```python
from build123d import *

# Parameters (mm, degrees)
BOSS_EXTRUDE1_DEPTH = 29.5
CUT_EXTRUDE1_DEPTH  = 27.5
SKETCH4_R           = 1.375
BOSS_EXTRUDE2_DEPTH = 6
CUT_EXTRUDE2_REACH  = 62
SKETCH5_W           = 8.5
SKETCH5_H           = 4
CUT_EXTRUDE3_REACH  = 64
SKETCH6_W           = 10
SKETCH6_H           = 6
BOSS_EXTRUDE3_DEPTH = 12
FILLET1_R           = 1


with BuildPart() as part:
    # Sketch1 → Boss-Extrude1 (new body)
    with BuildSketch(Plane(origin=(0, 0, 0), x_dir=(1, 0, 0), z_dir=(0, 1, 0))):
        with BuildLine():
            Line((-25, -31), (25, -31))
            ThreePointArc((25, -31), (28.535533906, -29.535533906), (30, -26))
            Line((30, -26), (30, 26))
            ThreePointArc((30, 26), (28.535533906, 29.535533906), (25, 31))
            Line((25, 31), (-25, 31))
            ThreePointArc((-25, 31), (-28.535533906, 29.535533906), (-30, 26))
            Line((-30, 26), (-30, -26))
            ThreePointArc((-30, -26), (-28.535533906, -29.535533906), (-25, -31))
        make_face()
    extrude(amount=BOSS_EXTRUDE1_DEPTH)

    # Sketch2 → Cut-Extrude1 (cut)
    with BuildSketch(Plane(origin=(0, 29.5, 0), x_dir=(1, 0, 0), z_dir=(0, 1, 0))):
        with BuildLine():
            Line((-25, -29), (25, -29))
            ThreePointArc((25, -29), (27.121320344, -28.121320344), (28, -26))
            Line((28, -26), (28, 26))
            ThreePointArc((28, 26), (27.121320344, 28.121320344), (25, 29))
            Line((25, 29), (-25, 29))
            ThreePointArc((-25, 29), (-27.121320344, 28.121320344), (-28, 26))
            Line((-28, 26), (-28, -26))
            ThreePointArc((-28, -26), (-27.121320344, -28.121320344), (-25, -29))
        make_face()
    extrude(amount=-CUT_EXTRUDE1_DEPTH, mode=Mode.SUBTRACT)

    # Sketch4 → Boss-Extrude2 (add)
    with BuildSketch(Plane(origin=(0, 2, 0), x_dir=(1, 0, 0), z_dir=(0, 1, 0))):
        with BuildLine():
            Line((-17.25, 23.25), (-17.25, 29))
            Line((-17.25, 29), (-25, 29))
            ThreePointArc((-25, 29), (-27.121320344, 28.121320344), (-28, 26))
            Line((-28, 26), (-28, 18.25))
            Line((-28, 18.25), (-22.25, 18.25))
            ThreePointArc((-22.25, 18.25), (-18.714466094, 19.714466094), (-17.25, 23.25))
        make_face()
        with Locations((-22.25, 23.25)):
            Circle(SKETCH4_R, mode=Mode.SUBTRACT)
        with BuildLine():
            Line((22.25, 18.25), (28, 18.25))
            Line((28, 18.25), (28, 26))
            ThreePointArc((28, 26), (27.121320344, 28.121320344), (25, 29))
            Line((25, 29), (17.25, 29))
            Line((17.25, 29), (17.25, 23.25))
            ThreePointArc((17.25, 23.25), (18.714466094, 19.714466094), (22.25, 18.25))
        make_face()
        with Locations((22.25, 23.25)):
            Circle(SKETCH4_R, mode=Mode.SUBTRACT)
        with BuildLine():
            Line((-25, -29), (-17.25, -29))
            Line((-17.25, -29), (-17.25, -23.25))
            ThreePointArc((-17.25, -23.25), (-18.714466094, -19.714466094), (-22.25, -18.25))
            Line((-22.25, -18.25), (-28, -18.25))
            Line((-28, -18.25), (-28, -26))
            ThreePointArc((-28, -26), (-27.121320344, -28.121320344), (-25, -29))
        make_face()
        with Locations((-22.25, -23.25)):
            Circle(SKETCH4_R, mode=Mode.SUBTRACT)
        with BuildLine():
            Line((28, -26), (28, -18.25))
            Line((28, -18.25), (22.25, -18.25))
            ThreePointArc((22.25, -18.25), (18.714466094, -19.714466094), (17.25, -23.25))
            Line((17.25, -23.25), (17.25, -29))
            Line((17.25, -29), (25, -29))
            ThreePointArc((25, -29), (27.121320344, -28.121320344), (28, -26))
        make_face()
        with Locations((22.25, -23.25)):
            Circle(SKETCH4_R, mode=Mode.SUBTRACT)
    extrude(amount=BOSS_EXTRUDE2_DEPTH)

    # Sketch5 → Cut-Extrude2 (cut, up to next)
    with BuildSketch(Plane.ZY.offset(30), mode=Mode.PRIVATE) as cut_extrude2_sk1:
        with Locations((-8.5, 18)):
            Rectangle(SKETCH5_W, SKETCH5_H)
    cut_extrude2_tool1 = extrude(cut_extrude2_sk1.sketch, amount=-CUT_EXTRUDE2_REACH, mode=Mode.PRIVATE) & part.part
    add(cut_extrude2_tool1.solids().sort_by_distance((-30, 18, -8.5))[0], mode=Mode.SUBTRACT)

    # Sketch6 → Cut-Extrude3 (cut, up to next)
    with BuildSketch(Plane(origin=(0, 0, -31), x_dir=(-1, 0, 0), z_dir=(0, 0, -1)), mode=Mode.PRIVATE) as cut_extrude3_sk1:
        with Locations((11.75, 19)):
            Rectangle(SKETCH6_W, SKETCH6_H)
    cut_extrude3_tool1 = extrude(cut_extrude3_sk1.sketch, amount=-CUT_EXTRUDE3_REACH, mode=Mode.PRIVATE) & part.part
    add(cut_extrude3_tool1.solids().sort_by_distance((-11.75, 19, -31))[0], mode=Mode.SUBTRACT)

    # Sketch7 → Boss-Extrude3 (add)
    with BuildSketch(Plane.ZY.offset(6)):
        Polygon((-29, 29.5), (-29, 26.5), (-27, 29.5), align=None)
    extrude(amount=-BOSS_EXTRUDE3_DEPTH)

    # Fillet1
    fillet1_edges = [part.edges().sort_by_distance(p)[0] for p in [
        (0, 0, -31),
        (28.535533906, 0, -29.535533906),
        (30, 0, 0),
        (28.535533906, 0, 29.535533906),
        (0, 0, 31),
        (-28.535533906, 0, 29.535533906),
        (-30, 0, 0),
        (-28.535533906, 0, -29.535533906),
    ]]
    fillet(fillet1_edges, radius=FILLET1_R)


solid = part.part
```
CAD build for the part. Positions are in the model's coordinates, mm. A direction names the side the tool comes from. Coordinates: 2 decimals unless noted, no trailing zeros. Order: outer loops, then holes, each group sorted by start corner. A loop starts at its lowest first (then second) coordinate and runs counter-clockwise, first axis right, second up.
(1) Saw through at C-C, the plane z = -11.5. Write the cut outline in (x, y), and give its area (3 significant figures).
Solution:
outline: (-30, 1) arc R1 ccw to (-29, 0) - (29, 0) arc R1 ccw to (30, 1) - (30, 29.5) - (28, 29.5) - (28, 2) - (-28, 2) - (-28, 16) - (-30, 16) - close; (-30, 20) - (-28, 20) - (-28, 29.5) - (-30, 29.5) - close
area: 222 mm2
(2) Drill centre lines: L1, parallel to Z at x = -22.25, y = 6.4 (3 decimals); L2, parallel to X at y = 4.25, z = 23.25 (3 decimals). Where is each one in solid material? Low to high.
Solution:
L1: z = -31 to -24.625, -21.875 to -18.25, 18.25 to 21.875, 24.625 to 31
L2: x = -30 to -23.625, -20.875 to -17.25, 17.25 to 20.875, 23.625 to 30
(3) Saw through at B-B, the plane y = 25.5. Write the cut outline in (x, z), and give its area (3 significant figures).
Solution:
outline: (-30, -26) arc R5 ccw to (-25, -31) - (25, -31) arc R5 ccw to (30, -26) - (30, 26) arc R5 ccw to (25, 31) - (-25, 31) arc R5 ccw to (-30, 26) - close; hole (-28, -26) arc R3 ccw to (-25, -29) - (25, -29) arc R3 ccw to (28, -26) - (28, 26) arc R3 ccw to (25, 29) - (-25, 29) arc R3 ccw to (-28, 26) - close
area: 458 mm2
(4) Saw through at A-A, the plane x = -8.5. Write the cut outline in (y, z), and give its area (3 significant figures).
Solution:
outline: (0, -30) arc R1 ccw to (1, -31) - (16, -31) - (16, -29) - (2, -29) - (2, 29) - (29.5, 29) - (29.5, 31) - (1, 31) arc R1 ccw to (0, 30) - close; (22, -31) - (29.5, -31) - (29.5, -29) - (22, -29) - close
area: 222 mm2
(5) Pin check, flat tips, straight feed: pin 1 Ø1.4 at (x, z) = (22, -23) entering from +Y; pin 2 Ø3 at (x, z) = (22.25, -23.25) entering from +Y; pin 3 Ø0.6 at (y, z) = (19, -30) entering from +X. Stop position of each tip, or through.
Solution:
pin 1: stops at y = 2
pin 2: stops at y = 8
pin 3: stops at x = 28.36
(6) Saw through at D-D, the plane y = 5. Write the cut outline in (x, z) (3 decimals), and give its area (3 significant figures).
Solution:
outline: (-30, -26) arc R5 ccw to (-25, -31) - (25, -31) arc R5 ccw to (30, -26) - (30, 26) arc R5 ccw to (25, 31) - (-25, 31) arc R5 ccw to (-30, 26) - close; hole (-28, -18.25) - (-22.25, -18.25) arc R5 cw to (-17.25, -23.25) - (-17.25, -29) - (17.25, -29) - (17.25, -23.25) arc R5 cw to (22.25, -18.25) - (28, -18.25) - (28, 18.25) - (22.25, 18.25) arc R5 cw to (17.25, 23.25) - (17.25, 29) - (-17.25, 29) - (-17.25, 23.25) arc R5 cw to (-22.25, 18.25) - (-28, 18.25) - close; hole circle Ø2.75 at (-22.25, -23.25); hole circle Ø2.75 at (-22.25, 23.25); hole circle Ø2.75 at (22.25, -23.25); hole circle Ø2.75 at (22.25, 23.25)
area: 868 mm2
(7) Which spindle directions (+Z, -Z, +X, -X, +Y, -Y) get a long thin tool onto all of the face, cutting with end or side? Do faces 3 (the face through (-12, 16, -30)), 4 (the face through (-25, 5, -18.25)), 5 (the face through (0, 15, 31)). Say none if no direction does.
Solution:
face 3: -Z
face 4: +Y
face 5: +Z, +X, -X, +Y, -Y
(8) Mould opens along Y. For faces 1 (the face through (-29, 18, -12.75)), 2 (the face through (-30, 15, 0)) say: released by +Y, released by -Y, zero draft, split by the parting line, or undercut.
Solution:
face 1: undercut
face 2: zero draft
